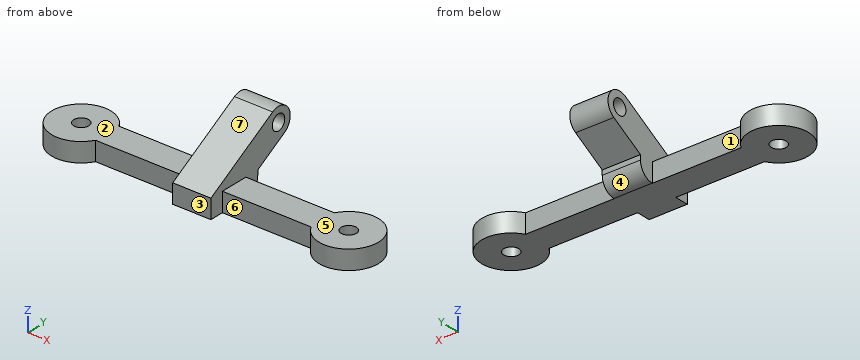
```python
from build123d import *

# Parameters (mm, degrees)
CROQUIS1_R                   = 1.6
SALIENTE_EXTRUIR1_DEPTH      = 4
CROQUIS2_R                   = 1.6
SALIENTE_EXTRUIR2_DEPTH      = 4
SALIENTE_EXTRUIR2_DEPTH_BACK = 4
REDONDEO1_R                  = 3


with BuildPart() as part:
    # Croquis1 → Saliente-Extruir1 (new body)
    with BuildSketch(Plane.XY):
        with BuildLine():
            Line((5.425863987, -3), (50.574136013, -3))
            ThreePointArc((50.574136013, -3), (62.2, 0), (50.574136013, 3))
            Line((50.574136013, 3), (5.425863987, 3))
            ThreePointArc((5.425863987, 3), (-6.2, 0), (5.425863987, -3))
        make_face()
        Circle(CROQUIS1_R, mode=Mode.SUBTRACT)
        with Locations((56, 0)):
            Circle(CROQUIS1_R, mode=Mode.SUBTRACT)
    extrude(amount=SALIENTE_EXTRUIR1_DEPTH)

    # Croquis2 → Saliente-Extruir2 (add, two sides)
    with BuildSketch(Plane(origin=(28, 0, 0), x_dir=(0, 0, -1), z_dir=(1, 0, 0))) as saliente_extruir2_sk:
        with BuildLine():
            Line((-4, -5.939790903), (-13.133231147, 9.879429481))
            ThreePointArc((-13.133231147, 9.879429481), (-12.035154935, 13.977505692), (-7.937078724, 12.879429481))
            Line((-7.937078724, 12.879429481), (-4, 6.060209097))
            Line((-4, 6.060209097), (0, 6.060209097))
            Line((0, 6.060209097), (0, -5.939790903))
            Line((0, -5.939790903), (-4, -5.939790903))
        make_face()
        with Locations((-10.535154935, 11.379429481)):
            Circle(CROQUIS2_R, mode=Mode.SUBTRACT)
    extrude(amount=SALIENTE_EXTRUIR2_DEPTH)
    extrude(saliente_extruir2_sk.sketch, amount=-SALIENTE_EXTRUIR2_DEPTH_BACK)

    # Redondeo1
    redondeo1_edges = [part.edges().sort_by_distance(p)[0] for p in [
        (28, 6.060209097, 0),
    ]]
    fillet(redondeo1_edges, radius=REDONDEO1_R)


solid = part.part
```
Work out the finished part from the listing and answer in its coordinate system (mm). Face numbers are marked on the shaded views. A direction names the side the tool comes from. Give positions to 0.01 mm unless a question says otherwise; leave off trailing zeros. Loops run counter-clockwise (first coordinate to the right, second up) from the corner with the lowest first, then second, coordinate; pieces in that order, holes last. Notation, with made-up numbers: (-24.5, 21) -> (-2.5, 21) arc R19 ccw to (-2.5, 47) -> close; hole circle Ø10 at (39, 81.5). An arc over 180 degrees is marked (long way). Write item = value, one per line. Start each with the question number.
(1) Given pin 1 Ø8 at (x, y) = (41.5, 2.5) entering from -Z; pin 2 Ø4.5 at (x, z) = (17.5, 1.5) entering from -Y; pin 3 Ø4.5 at (x, z) = (40.5, 2.5) entering from +Y; pin 4 Ø0.5 at (x, z) = (29, 3.5) entering from +Y, each flat-ended and moving along its own axis, determine where each tip first touches the part or whether it passes through.
(2) Which of the six approach directions +Z, -Z, +X, -X, +Y, -Y give full straight-line access (tool end or side, diameter ignored) to the marked faces 1, 2, 3, 4 and 5?
(3) Find the intervals of material crossed by probe 1 along Y at (x, z) = (0, 2.2); probe 2 along X at (y, z) = (-0.5, 6.5); probe 3 along Y at (x, z) = (20.5, 3.5), in increasing order. Write a range as from..to.
(4) Find section C-C on y = 0. Give the vertices of the cut face in (x, z).
(5) The mould has two halves that part along X. Classify the marked faces 6 and 7: +X half, -X half, draft (parallel to the pull), parting line (faces both ways), or undercut.
(6) Find section D-D on y = 7. Give the vertices of the cut face in (x, z), and give its area (3 significant figures).
(7) Find section A-A on x = 0. Give the vertices of the cut face in (y, z), and give its area (3 significant figures).
(8) Find section B-B on z = 10.75. Give the vertices of the cut face in (x, y), and give its area (3 significant figures).
From the geometry:
q1.pin_1 = 0
q1.pin_2 = -3
q1.pin_3 = 3
q1.pin_4 = 6.06
q2.face_1 = +Z, -Z, +Y
q2.face_2 = +Z, -X, +Y, -Y
q2.face_3 = +Z, -Z, -Y
q2.face_4 = -Z, +Y
q2.face_5 = +Z, +X, +Y, -Y
q3.probe_1 = -6.2..-1.6, 1.6..6.2
q3.probe_2 = 24..32
q3.probe_3 = -3..3
q4.outline = (-6.2, 0) -> (-1.6, 0) -> (-1.6, 4) -> (-6.2, 4) -> close; (1.6, 0) -> (54.4, 0) -> (54.4, 4) -> (32, 4) -> (32, 7.43) -> (24, 7.43) -> (24, 4) -> (1.6, 4) -> close; (57.6, 0) -> (62.2, 0) -> (62.2, 4) -> (57.6, 4) -> close
q5.face_6 = undercut
q5.face_7 = draft
q6.outline = (24, 4.54) -> (32, 4.54) -> (32, 11.47) -> (24, 11.47) -> close
q6.area = 55.4 mm^2
q7.outline = (-6.2, 0) -> (-1.6, 0) -> (-1.6, 4) -> (-6.2, 4) -> close; (1.6, 0) -> (6.2, 0) -> (6.2, 4) -> (1.6, 4) -> close
q7.area = 36.8 mm^2
q8.outline = (24, 5.75) -> (32, 5.75) -> (32, 9.79) -> (24, 9.79) -> close; (24, 12.96) -> (32, 12.96) -> (32, 14.37) -> (24, 14.37) -> close
q8.area = 43.6 mm^2
